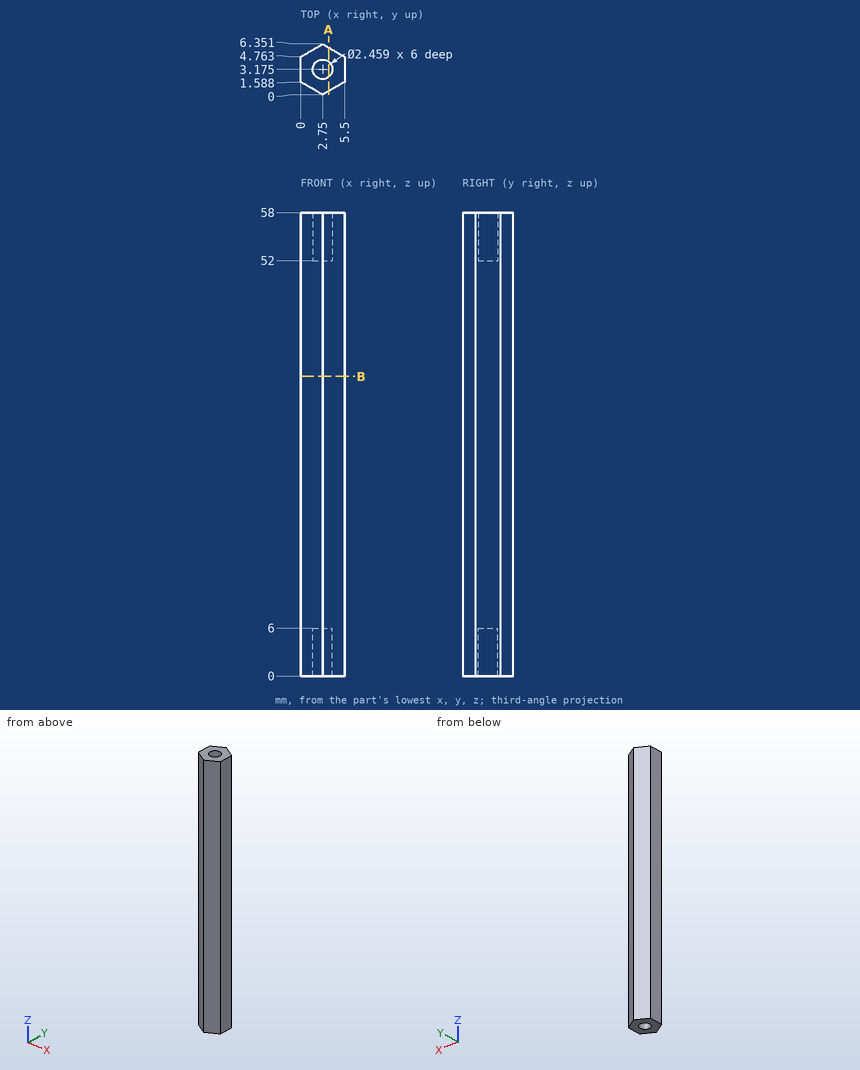
Answer from the drawing. Dimensions are ordinates in mm from the lowest x, y and z of the part. Round coordinates to 2 decimals unless told otherwise and drop trailing zeros. Loops run counter-clockwise (first coordinate to the right, second up) from the corner with the lowest first, then second, coordinate; pieces in that order, holes last. Notation, with made-up numbers: (82, 39.5) - (109, 39.5) arc R33 cw to (109, 77.5) - close; hole circle Ø5 at (-24.75, 1.25). An arc over 180 degrees is marked (long way). Return JSON: item names as keys, results as strings. Group by question number.
1. The part is cut by section B-B on z = 37.5. Determine the outline of the cut face in (x, y).
2. Each of these flat-tipped pins is pushed along its axis until it touches: P1, Ø2.5, axis at x = 3, y = 3, coming from the -Z side; P2, Ø1.5, axis at x = 2.75, y = 3.18, coming from the -Z side; P3, Ø3, axis at x = 3.5, z = 25, coming from the +Y side. Where does it stop, or does it pass through?
3. The part is cut by section A-A on x = 3.5. Determine the outline of the cut face in (y, z), then the cut area to 3 significant figures.
4. Consider probe 1 along Z at (x, y) = (2.05, 2.75); probe 2 along Y at (x, z) = (1.35, 8.5); probe 3 along X at (y, z) = (6.25, 34) (1 decimal). Determine where each line is inside the solid, lowest interval first.
Resolved:
{
 "1": {"outline": "(0, 1.59) - (2.75, 0) - (5.5, 1.59) - (5.5, 4.76) - (2.75, 6.35) - (0, 4.76) - close"},
 "2": {"P1": "stops at z = 0", "P2": "stops at z = 6", "P3": "stops at y = 6.35"},
 "3": {"outline": "(0.43, 0) - (2.2, 0) - (2.2, 6) - (4.15, 6) - (4.15, 0) - (5.92, 0) - (5.92, 58) - (4.15, 58) - (4.15, 52) - (2.2, 52) - (2.2, 58) - (0.43, 58) - close", "area": "295 mm²"},
 "4": {"probe 1": "z = 6 to 52", "probe 2": "y = 0.81 to 5.54", "probe 3": "x = 2.6 to 2.9"}
}
